Could you check a few things on this drawing? It's one solid part, dimensions in mm from its lowest x, y, z. A direction names the side the tool comes from. Give positions to 0.01 mm unless a question says otherwise; leave off trailing zeros. Loops run counter-clockwise (first coordinate to the right, second up) from the corner with the lowest first, then second, coordinate; pieces in that order, holes last. Notation, with made-up numbers: (51, -8.5) - (100, -8.5) arc R22 cw to (100, 26.5) - close; hole circle Ø6 at (54.25, 34). An arc over 180 degrees is marked (long way). Put each result on its own line as item: value. Start each with the question number.
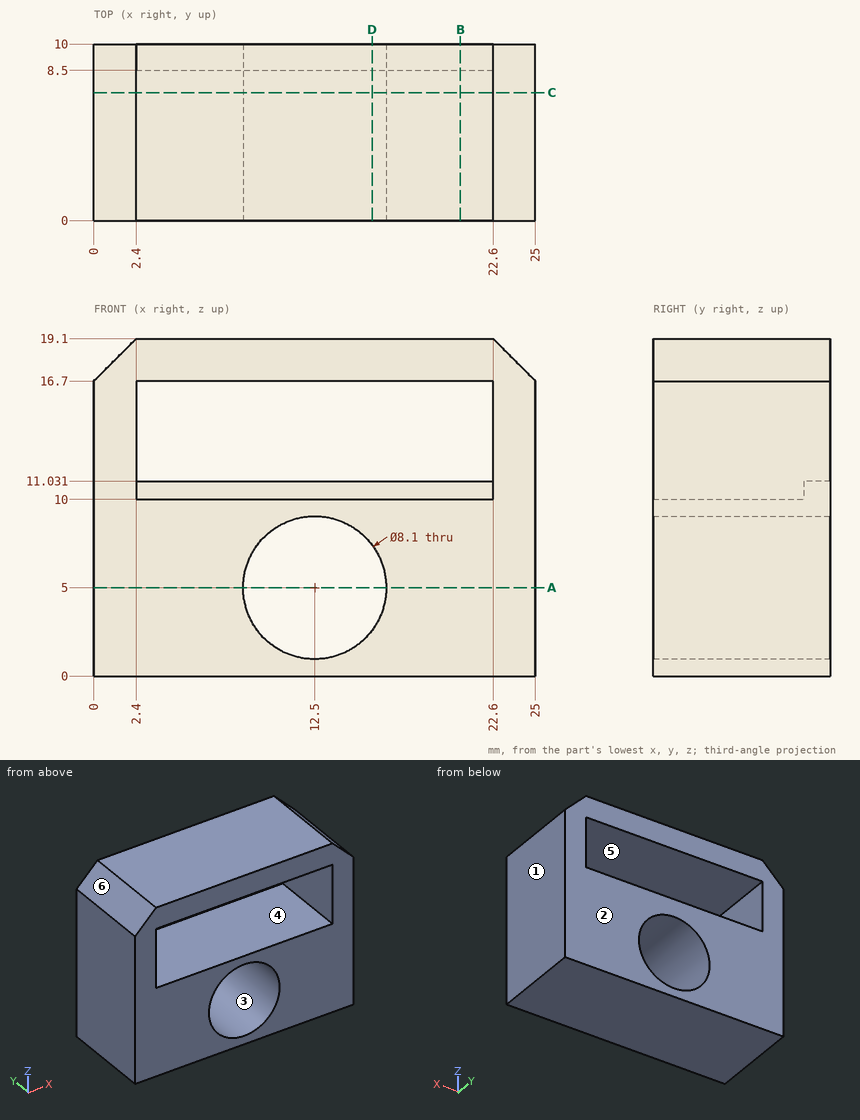
1) Suppose I cut it at A-A on z = 5. Please give me the cut outline in (x, y).
2) Suppose I cut it at B-B on x = 20.75. Please give me the cut outline in (y, z), plus the area to 3 significant figures.
3) Thinking about a two-plate mould opening in X: for the marked faces 1, 2 and 3, which applies, pulls with the +X half, pulls with the -X half, needs draft (parallel to the pull), parting line crosses it, or undercut?
4) Suppose I cut it at C-C on y = 7.25. Please give me the cut outline in (x, z), plus the area to 3 significant figures.
5) Suppose I cut it at D-D on x = 15.75. Please give me the cut outline in (y, z), plus the area to 3 significant figures.
6) Which directions (+Z, -Z, +X, -X, +Y, -Y) give clear straight access to the entire face, cutting with the end or side of a thin tool? Please do the marked faces 4, 5 and 6.
7) I need wall thicknesses on line 1 (Z direction, x = 2.75, y = 1.5); line 2 (X direction, y = 2.75, z = 5); line 3 (Z direction, x = 11.5, y = 9.25) (1 decimal). Which ranges of each line are inside material? Lowest first, please.
8) I'm going to push a flat-ended pin straight in: P1, Ø5, axis at y = 4.5, z = 16, coming from the -X side. Where does the tip first touch, or does it pass through?
Ans:
1. outline: (0, 0) - (8.45, 0) - (8.45, 10) - (0, 10) - close; (16.55, 0) - (25, 0) - (25, 10) - (16.55, 10) - close
2. outline: (0, 0) - (10, 0) - (10, 11.03) - (8.5, 11.03) - (8.5, 10) - (0, 10) - close; (0, 16.7) - (10, 16.7) - (10, 19.1) - (0, 19.1) - close
2. area: 126 mm²
3. face 1: pulls with the +X half
3. face 2: needs draft
3. face 3: undercut
4. outline: (0, 0) - (25, 0) - (25, 16.7) - (22.6, 19.1) - (2.4, 19.1) - (0, 16.7) - close; hole (2.4, 10) - (22.6, 10) - (22.6, 16.7) - (2.4, 16.7) - close; hole circle Ø8.1 at (12.5, 5)
4. area: 285 mm²
5. outline: (0, 0) - (10, 0) - (10, 2.58) - (0, 2.58) - close; (0, 7.42) - (10, 7.42) - (10, 11.03) - (8.5, 11.03) - (8.5, 10) - (0, 10) - close; (0, 16.7) - (10, 16.7) - (10, 19.1) - (0, 19.1) - close
5. area: 77.2 mm²
6. face 4: -Y
6. face 5: +Y, -Y
6. face 6: +Z, -X, +Y, -Y
7. line 1: z = 0 to 10, 16.7 to 19.1
7. line 2: x = 0 to 8.45, 16.55 to 25
7. line 3: z = 0 to 1.1, 8.9 to 11, 16.7 to 19.1
8. P1: stops at x = 0
